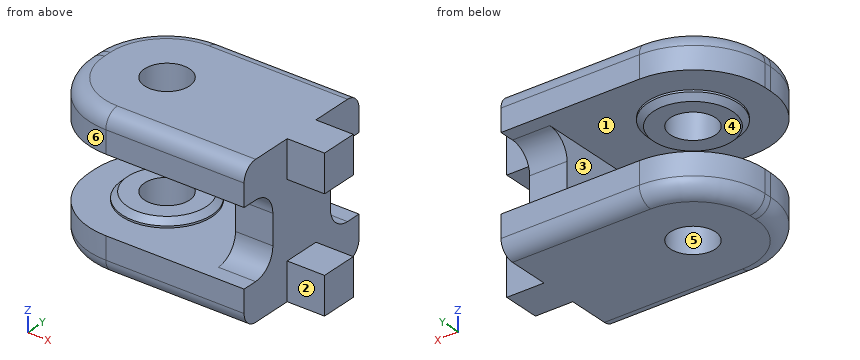
```python
from build123d import *

# Parameters (mm, degrees)
BOX007_W          = 11
BOX007_H          = 7
BOX007_DEPTH      = 10
FILLET_R          = 3
ARRAY_COUNT       = 2
ARRAY_ANGLE       = 180
CYLINDER004_R     = 3
CYLINDER004_DEPTH = 30
CYLINDER005_R     = 6
CYLINDER005_DEPTH = 4
BOX005_W          = 23
BOX005_H          = 20
BOX005_DEPTH      = 5
BOX003_W          = 10
BOX003_H          = 5
BOX003_DEPTH      = 5
BOX004_W          = 10
BOX004_H          = 5
BOX004_DEPTH      = 5
BOX_W             = 5
BOX_H             = 20
BOX_DEPTH         = 20
BOX006_W          = 23
BOX006_H          = 20
BOX006_DEPTH      = 5
CYLINDER006_R     = 6
CYLINDER006_DEPTH = 4
CHAMFER_SIZE      = 0.75
CHAMFER001_SIZE   = 0.75
FILLET001_R       = 9.5
FILLET002_R       = 2


with BuildPart() as array:
    # Box007 → Box007 (new body)
    with BuildSketch(Plane(origin=(10, 5, -5), x_dir=(1, 0, 0), z_dir=(0, 0, 1))):
        with Locations((5.5, 3.5)):
            Rectangle(BOX007_W, BOX007_H)
    extrude(amount=BOX007_DEPTH)


with BuildPart() as array_1:
    # BaseFeature placement: moved
    add(array.part.moved(Location((-10, -5, 5))))

    # Fillet
    fillet_edges = [array_1.edges().sort_by_distance(p)[0] for p in [
        (5.5, 0, 10),
        (5.5, 0, 0),
    ]]
    fillet(fillet_edges, radius=FILLET_R)


with BuildPart() as array_2:
    # Body placement: moved
    add(array_1.part.moved(Location((-5, 5, 0))))

    # Array: Array ×2 about axis
    array_axis = Axis((0, 0, 0), (0, 0, 1))


with BuildPart() as array_3:
    add(array_2.part)
    for i in range(1, ARRAY_COUNT):
        add(array_2.part.rotate(array_axis, i * ARRAY_ANGLE / (ARRAY_COUNT - 1)))


with BuildPart() as array_4:
    # Array placement: moved
    add(array_3.part.moved(Location((14, 0, -5))))


with BuildPart() as cilindro004:
    # Cylinder004 → Cylinder004 (new body)
    with BuildSketch(Plane.XY.offset(-15)):
        Circle(CYLINDER004_R)
    extrude(amount=CYLINDER004_DEPTH)


with BuildPart() as obj1:
    # Cylinder005 → Cylinder005 (new body)
    with BuildSketch(Plane.XY.offset(-8)):
        Circle(CYLINDER005_R)
    extrude(amount=CYLINDER005_DEPTH)


with BuildPart() as cubo:
    # Box005 → Box005 (new body)
    with BuildSketch(Plane(origin=(-10, -10, -10), x_dir=(1, 0, 0), z_dir=(0, 0, 1))):
        with Locations((11.5, 10)):
            Rectangle(BOX005_W, BOX005_H)
    extrude(amount=BOX005_DEPTH)


with BuildPart() as cubo002:
    # Box003 → Box003 (new body)
    with BuildSketch(Plane(origin=(13, -2.5, 5), x_dir=(1, 0, 0), z_dir=(0, 0, 1))):
        with Locations((5, 2.5)):
            Rectangle(BOX003_W, BOX003_H)
    extrude(amount=BOX003_DEPTH)


with BuildPart() as cubo003:
    # Box004 → Box004 (new body)
    with BuildSketch(Plane(origin=(13, -2.5, -10), x_dir=(1, 0, 0), z_dir=(0, 0, 1))):
        with Locations((5, 2.5)):
            Rectangle(BOX004_W, BOX004_H)
    extrude(amount=BOX004_DEPTH)


with BuildPart() as fusion002001:
    # Box → Box (new body)
    with BuildSketch(Plane(origin=(13, -10, -10), x_dir=(1, 0, 0), z_dir=(0, 0, 1))):
        with Locations((2.5, 10)):
            Rectangle(BOX_W, BOX_H)
    extrude(amount=BOX_DEPTH)

    # Fusion002: union Cubo002, Cubo003
    add(cubo002.part)
    add(cubo003.part)


with BuildPart() as fusion002002001:
    # Box006 → Box006 (new body)
    with BuildSketch(Plane(origin=(-10, -10, 5), x_dir=(1, 0, 0), z_dir=(0, 0, 1))):
        with Locations((11.5, 10)):
            Rectangle(BOX006_W, BOX006_H)
    extrude(amount=BOX006_DEPTH)

    # Fusion002002: union Cubo, Fusion002001
    add(cubo.part)
    add(fusion002001.part)


with BuildPart() as body001:
    # Cylinder006 → Cylinder006 (new body)
    with BuildSketch(Plane.XY.offset(4)):
        Circle(CYLINDER006_R)
    extrude(amount=CYLINDER006_DEPTH)

    # Fusion002002002: union obj1, Fusion002002001
    add(obj1.part)
    add(fusion002002001.part)

    # Cut001: cut Cilindro004
    add(cilindro004.part, mode=Mode.SUBTRACT)

    # Cut002: cut Array
    add(array_4.part, mode=Mode.SUBTRACT)

    # Chamfer
    chamfer_edges = [body001.edges().sort_by_distance(p)[0] for p in [
        (-6, 0, -4),
    ]]
    chamfer(chamfer_edges, length=CHAMFER_SIZE)

    # Chamfer001
    chamfer001_edges = [body001.edges().sort_by_distance(p)[0] for p in [
        (-6, 0, 4),
    ]]
    chamfer(chamfer001_edges, length=CHAMFER001_SIZE)

    # Fillet001
    fillet001_edges = [body001.edges().sort_by_distance(p)[0] for p in [
        (-10, 10, 7.5),
        (-10, -10, 7.5),
        (-10, -10, -7.5),
        (-10, 10, -7.5),
    ]]
    fillet(fillet001_edges, radius=FILLET001_R)

    # Fillet002
    fillet002_edges = [body001.edges().sort_by_distance(p)[0] for p in [
        (8.75, 10, 10),
        (8.75, 10, -10),
    ]]
    fillet(fillet002_edges, radius=FILLET002_R)


solid = body001.part
```
Here's how the part is built. I have some questions about the finished solid (model axes, mm). Face numbers are marked on the shaded views. A direction names the side the tool comes from. Round coordinates to 2 decimals unless told otherwise and drop trailing zeros. Order: outer loops, then holes, each group sorted by start corner. A loop starts at its lowest first (then second) coordinate and runs counter-clockwise, first axis right, second up. Notation, with made-up numbers: M -8.75,-32 L 6.25,-32 A27 cw 6.25,0 Z; hole C 50,75.5 d6. An arc over 180 degrees is marked long. One line per question, with ' | ' between items.
1) I want a section at D-D, the plane x = 6.5. Write out the boundary of the cut face in (y, z), then the cut area to 3 significant figures.
Working result:
outline: M -10,-8 A2 ccw -8,-10 L 8,-10 A2 ccw 10,-8 L 10,-5 L -10,-5 Z; M -10,5 L 10,5 L 10,8 A2 ccw 8,10 L -8,10 A2 ccw -10,8 Z | area: 197 mm²
2) I want a section at C-C, the plane z = 5.75. Write out the boundary of the cut face in (x, y), then the cut area to 3 significant figures.
Working result:
outline: M -10,-0.5 A9.5 ccw -0.5,-10 L 18,-10 L 18,-2.5 L 23,-2.5 L 23,2.5 L 18,2.5 L 18,10 L -0.5,10 A9.5 ccw -10,0.5 Z; hole C 0,0 d6 | area: 518 mm²
3) If we mould it in two halves opening along Y, with no side actions, what happens to the marked faces 4, 5 and 6? For each: +Y half, -Y half, draft (parallel to the pull), parting line (faces both ways), or undercut.
Working result:
face 4: draft | face 5: undercut | face 6: -Y half
4) I need wall thicknesses on line 1 along Y through (x, z) = (0, 6.25); line 2 along X through (y, z) = (0, 5.95); line 3 along Z through (x, y) = (21.5, -0.25). Which ranges of each line are inside material? Lowest first, please.
Working result:
line 1: -10 to -3, 3 to 10 | line 2: -10 to -3, 3 to 23 | line 3: -10 to -5, 5 to 10
5) For pin 1 Ø1.5 at (x, z) = (20.5, -8.5) entering from -Y; pin 2 Ø4 at (x, z) = (21, 7) entering from +Y; pin 3 Ø4.5 at (x, z) = (15.5, -0.5) entering from -Y; pin 4 Ø5 at (y, z) = (1, -3) entering from +X, each with a flat end and sliding along its axis, tell me the tip position at first contact or that it passes through.
Working result:
pin 1: y = -2.5 | pin 2: y = 2.5 | pin 3: y = -5.1 | pin 4: x = 23
6) I want a section at A-A, the plane y = 0. State how many separate pieces and enclosed holes the cut face has, then the cut area to 3 significant figures.
Working result:
separate pieces: 3 | enclosed holes: 0 | area: 329 mm²
7) For the marked faces 1, 2 and 3, which set-ups out of +Z, -Z, +X, -X, +Y, -Y let a thin tool reach every point of the face, with its end or its side?
Working result:
face 1: none | face 2: +Z, -Z, +X, -Y | face 3: +Y, -Y
